Here's how the part is built. I have some questions about the finished solid (model axes, mm). Face numbers are marked on the shaded views. Coordinates: 2 decimals unless noted, no trailing zeros. Write each loop counter-clockwise with the first axis right and the second up, starting at its lowest first coordinate (ties: lowest second). Pieces come first, ordered by that corner, then holes. Notation, with made-up numbers: (-22, 36) -> (28, 36) arc R21 ccw to (28, 56) -> close; hole circle Ø6 at (-20.5, -39). An arc over 180 degrees is marked (long way). Use a Markdown table: item, result. Add a question column.
Item 1: If I drill on line 1 along X through (y, z) = (310.5, 750.5); line 2 along Y through (x, z) = (-125.5, 465); line 3 along Y through (x, z) = (-22.5, 36.5), over which ranges is the centre line in solid material (lowest first)? Write a range as from..to.
Item 2: Imagine slicing it at B-B, the plane y = 432. Write out the boundary of the cut face in (x, z), and give its area (3 significant figures).
Item 3: Imagine slicing it at A-A, the plane z = 407.5. Write out the boundary of the cut face in (x, y).
Item 4: Imagine slicing it at C-C, the plane x = -35. Write out the boundary of the cut face in (y, z).
Item 5: If we mould it in two halves opening along Z, with no side actions, what happens to the marked faces 1, 2 and 3? For each: pulls with the +Z half, pulls with the -Z half, needs draft (parallel to the pull), parting line crosses it, or undercut.
Item 6: Will these pins go through, and if not, where does the flat tip stop? pin 1 Ø23.5 at (y, z) = (660.5, 416.5) entering from +X; pin 2 Ø6 at (y, z) = (589.5, 276.5) entering from -X; pin 3 Ø1 at (y, z) = (515.5, 83.5) entering from +X.
```python
from build123d import *

# Parameters (mm, degrees)
F1_DEPTH = 800


with BuildPart() as f1:
    # F0 (on Top) → F1 (new body)
    with BuildSketch(Plane.XY):
        Polygon((-89.048881, 0), (0, 0), (0, 499.227196), (-89.048881, 616.271885), align=None)
        Polygon((-98.031923, 0), (-89.048881, 0), (-89.048881, 616.271885), (-89.048881, 695.234752), (-98.031923, 700), (-98.031923, 699.936681), align=None)
        with BuildLine():
            Line((-120, 0), (-98.031923, 0))
            Line((-98.031923, 0), (-98.031923, 699.936681))
            ThreePointArc((-98.031923, 699.936681), (-108.294154, 693.949508), (-120, 691.916585))
            Line((-120, 691.916585), (-120, 0))
        make_face()
        with BuildLine():
            Line((-240, 0), (-120, 0))
            Line((-120, 0), (-120, 691.916585))
            ThreePointArc((-120, 691.916585), (-145.462987, 661.509664), (-166.336656, 627.786756))
            ThreePointArc((-166.336656, 627.786756), (-220.911757, 496.452626), (-240, 355.517413))
            Line((-240, 355.517413), (-240, 350))
            Line((-240, 350), (-240, 0))
        make_face()
        with BuildLine():
            ThreePointArc((-240, 355.517413), (-240.006916, 352.758707), (-240, 350))
            Line((-240, 350), (-240, 355.517413))
        make_face()
    extrude(amount=F1_DEPTH)


solid = f1.part
```
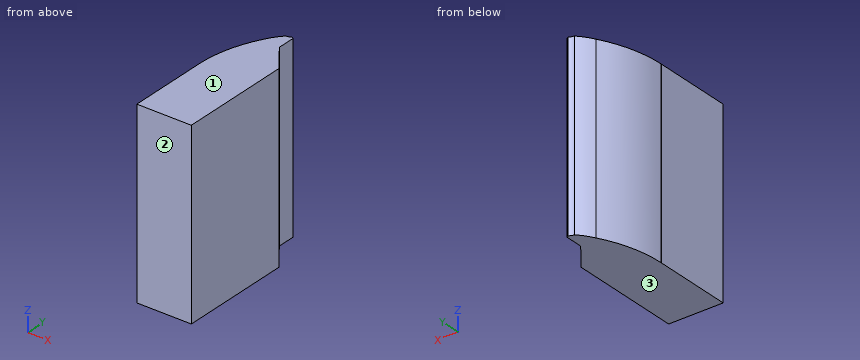
Ans:
| question | item | result |
|---|---|---|
| 1 | line 1 | x = -240..0 |
| 1 | line 2 | y = 0..686.06 |
| 1 | line 3 | y = 0..528.8 |
| 2 | outline | (-234.27, 0) -> (0, 0) -> (0, 800) -> (-234.27, 800) -> close |
| 2 | area | 187,000 mm^2 |
| 3 | outline | (-240, 0) -> (0, 0) -> (0, 499.23) -> (-89.05, 616.27) -> (-89.05, 695.23) -> (-98.03, 700) -> (-98.03, 699.94) arc R33.53 cw to (-120, 691.92) arc R277.81 ccw to (-166.34, 627.79) arc R550.21 ccw to (-240, 355.52) arc R550.21 ccw to (-240, 350) -> close |
| 4 | outline | (0, 0) -> (545.23, 0) -> (545.23, 800) -> (0, 800) -> close |
| 5 | face 1 | pulls with the +Z half |
| 5 | face 2 | needs draft |
| 5 | face 3 | pulls with the -Z half |
| 6 | pin 1 | stops at x = -89.05 |
| 6 | pin 2 | stops at x = -187.89 |
| 6 | pin 3 | stops at x = -12 |
